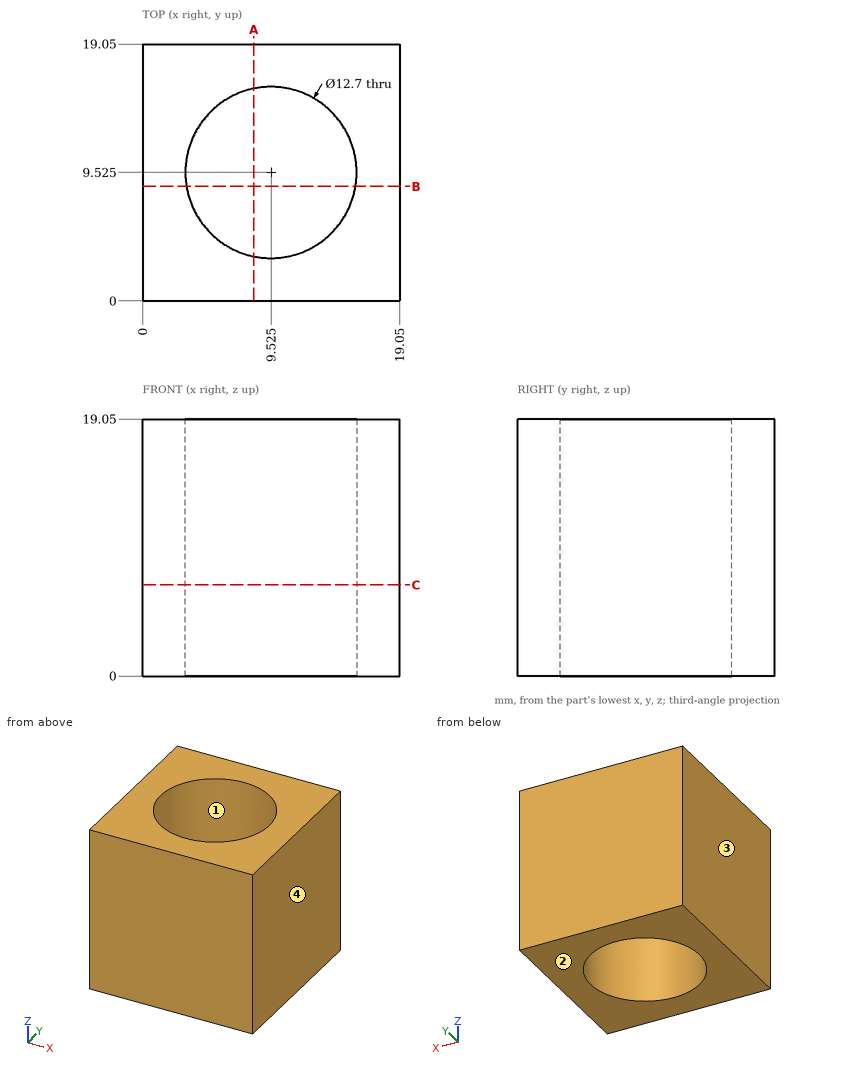
Geometry: see drawing. Coordinates: mm, zero at the bounding-box minimum. Coordinates: 2 decimals unless noted, no trailing zeros. Order: outer loops, then holes, each group sorted by start corner. A loop starts at its lowest first (then second) coordinate and runs counter-clockwise, first axis right, second up. Notation, with made-up numbers: (-25, 5.25) - (14, 5.25) arc R13 ccw to (14, 25.25) - close; hole circle Ø7 at (50.25, 67). An arc over 180 degrees is marked (long way). Use one line per item in the form item = value.
1) Section B-B (y = 8.5). Return loops of the section in (x, z), then the cut area to 3 significant figures.
Solutions:
outline = (0, 0) - (3.26, 0) - (3.26, 19.05) - (0, 19.05) - close; (15.79, 0) - (19.05, 0) - (19.05, 19.05) - (15.79, 19.05) - close
area = 124 mm^2
2) Section C-C (z = 6.75). Return loops of the section in (x, y) (3 decimals), then the cut area to 3 significant figures.
Solutions:
outline = (0, 0) - (19.05, 0) - (19.05, 19.05) - (0, 19.05) - close; hole circle Ø12.7 at (9.525, 9.525)
area = 236 mm^2
3) Ray query, L1, parallel to X at y = 9.75, z = 12.5; L2, parallel to Y at x = 7.5, z = 5; L3, parallel to Y at x = 7.75, z = 17. Return the intervals inside material, ascending.
Solutions:
L1 = 0 to 3.18, 15.87 to 19.05
L2 = 0 to 3.51, 15.54 to 19.05
L3 = 0 to 3.43, 15.62 to 19.05
4) Mould query, pull axis X, two halves, no side actions, for the marked faces 1, 2, 3 and 4. Classes: +X half, -X half, draft (parallel to the pull), parting line (faces both ways), or undercut.
Solutions:
face_1 = undercut
face_2 = draft
face_3 = -X half
face_4 = +X half
5) Section A-A (x = 8.25). Return loops of the section in (y, z), then the cut area to 3 significant figures.
Solutions:
outline = (0, 0) - (3.3, 0) - (3.3, 19.05) - (0, 19.05) - close; (15.75, 0) - (19.05, 0) - (19.05, 19.05) - (15.75, 19.05) - close
area = 126 mm^2
